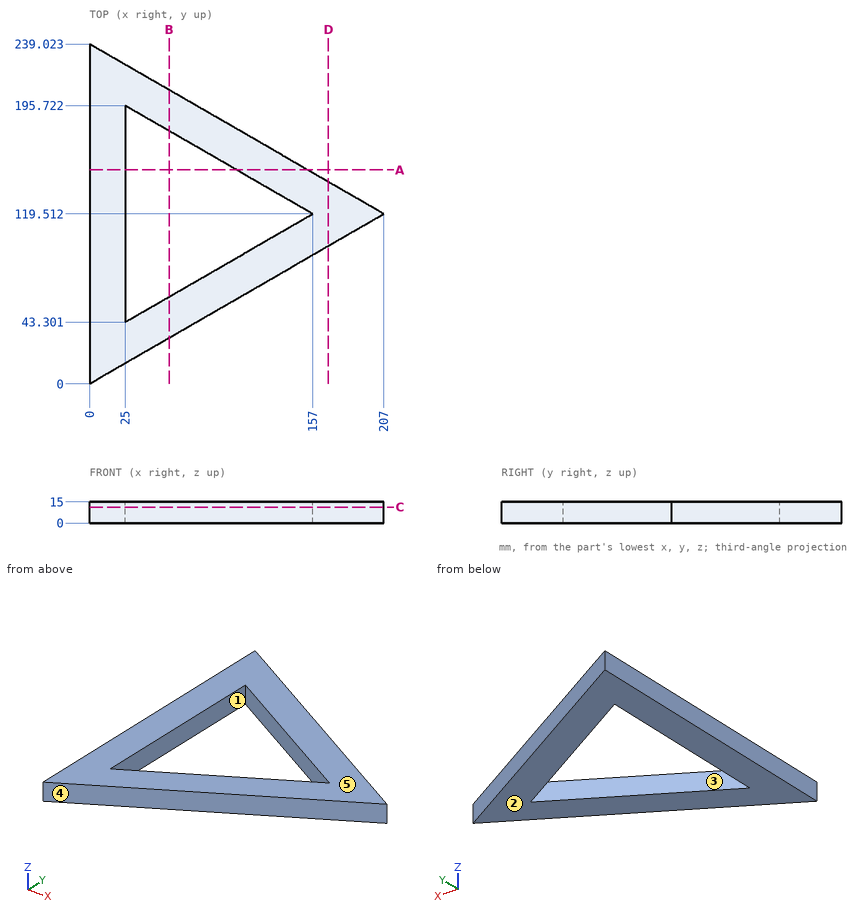
Geometry check sheet. Reference: drawing and pictorial views, mm from the part's lowest x, y, z. A direction names the side the tool comes from. Round coordinates to 2 decimals unless told otherwise and drop trailing zeros. Loops run counter-clockwise (first coordinate to the right, second up) from the corner with the lowest first, then second, coordinate; pieces in that order, holes last.
1. Sectioned sample at C-C on z = 11.25. Record the boundary of the cut face in (x, y).
2. Sectioned sample at B-B on x = 56. Record the boundary of the cut face in (y, z).
3. Scan lines: probe 1 along Y at (x, z) = (95.5, 7) (1 decimal); probe 2 along Y at (x, z) = (96, 1) (1 decimal); probe 3 along X at (y, z) = (173, 7.75) (1 decimal). Record each from-to range of solid material in increasing order.
4. Gauge pin test, flat ends, axial feed: pin 1 Ø2 at (x, z) = (58.5, 10.5) entering from +Y (1 decimal); pin 2 Ø1.5 at (x, z) = (122, 12) entering from +Y; pin 3 Ø4 at (x, z) = (54.5, 13.5) entering from +Y. Record the tip position at first contact, or that the pin passes through.
5. Sectioned sample at D-D on x = 168. Record the boundary of the cut face in (y, z) (1 decimal).
6. Set-up check for the marked faces 1 and 2: record each of +Z, -Z, +X, -X, +Y, -Y from which the full face is reachable in a straight line by a thin tool's end or side.
7. Sectioned sample at A-A on y = 150.5. Record the boundary of the cut face in (x, z).
8. Mould release check, pull along Y, two halves, no side actions. Record for the marked faces 3, 4 and 5: released by +Y, released by -Y, zero draft, split by the parting line, or undercut.
Recorded:
1. outline: (0, 0) - (207, 119.51) - (0, 239.02) - close; hole (25, 43.3) - (157, 119.51) - (25, 195.72) - close
2. outline: (32.33, 0) - (61.2, 0) - (61.2, 15) - (32.33, 15) - close; (177.82, 0) - (206.69, 0) - (206.69, 15) - (177.82, 15) - close
3. probe 1: y = 55.1 to 84, 155 to 183.9
3. probe 2: y = 55.4 to 84.3, 154.7 to 183.6
3. probe 3: x = 0 to 25, 64.4 to 114.4
4. pin 1: stops at y = 205.8
4. pin 2: stops at y = 169.02
4. pin 3: stops at y = 208.71
5. outline: (97, 0) - (142, 0) - (142, 15) - (97, 15) - close
6. face 1: +Z, -Z
6. face 2: -Z, +X, -X, +Y, -Y
7. outline: (0, 0) - (25, 0) - (25, 15) - (0, 15) - close; (103.33, 0) - (153.33, 0) - (153.33, 15) - (103.33, 15) - close
8. face 3: undercut
8. face 4: released by -Y
8. face 5: zero draft
